Source: CAD feature listing. Evaluate the final solid. Frame: model axes, mm. A direction names the side the tool comes from. Give positions to 0.01 mm unless a question says otherwise; leave off trailing zeros. Order: outer loops, then holes, each group sorted by start corner. A loop starts at its lowest first (then second) coordinate and runs counter-clockwise, first axis right, second up. Notation, with made-up numbers: M 32.5,5 L 74.5,5 A21 ccw 74.5,12 Z; hole C 86,36.5 d7. An arc over 180 degrees is marked long. Answer in a Markdown table with one row per item. Add a question column.
(1) Section query C-C, the plane z = 9. Return loops of the section in (x, y).
(2) Set-up query: faces 1 (the face through (-0.5, 6.5, 4.9)), 2 (the face through (5, 0, 5)). Return all of +Z, -Z, +X, -X, +Y, -Y with unobstructed straight access to the full face (end or side cutting, diameter ignored); none if empty.
(3) Pin query (flat end, axial travel): P1, Ø3, axis at y = 4, z = 4.5, coming from the +X side. Return the tip coordinate at first contact, or that it passes through.
(4) Mould query, pull axis Z, two halves, no side actions, for faces 3 (the face through (-0.507, 3.26, 6.983)), 4 (the face through (-1, 1, 4)). Classes: pulls with the +Z half, pulls with the -Z half, needs draft (parallel to the pull), parting line crosses it, or undercut.
(5) Section query B-B, the plane z = 5. Return loops of the section in (x, y).
(6) Material intervals for line 1 along Z through (x, y) = (-0.7, 3); line 2 along X through (y, z) = (0.25, 2.5), sorted ascending.
(7) Section query A-A, the plane y = 3. Return loops of the section in (x, z).
(8) Section query D-D, the plane y = 4.25. Return loops of the section in (x, z), plus the area to 3 significant figures.
from build123d import *

# Parameters (mm, degrees)
AUFSATZ_LINEAR_AUSTRAGEN1_DEPTH = 10
SKIZZE2_R                       = 2
SCHNITT_LINEAR_AUSTRAGEN1_DEPTH = 16.564382416


with BuildPart() as part:
    # Skizze1 → Aufsatz-Linear austragen1 (new body)
    with BuildSketch(Plane.XY):
        Polygon((0, 0), (0, 6.5), (-1, 6.5), (-1, -1), (9, -1), (9, 0), align=None)
    extrude(amount=AUFSATZ_LINEAR_AUSTRAGEN1_DEPTH)

    # Skizze2 → Schnitt-Linear austragen1 (cut, through all)
    with BuildSketch(Plane.ZY.offset(1)):
        with Locations(Location((5, 3, 0), (0, 0, 270))):
            Circle(SKIZZE2_R)
    extrude(amount=-SCHNITT_LINEAR_AUSTRAGEN1_DEPTH, mode=Mode.SUBTRACT)


solid = part.part
Values follow:
| question | item | result |
|---|---|---|
| 1 | outline | M -1,-1 L 9,-1 L 9,0 L 0,0 L 0,6.5 L -1,6.5 Z |
| 2 | face 1 | +Z, -Z, +X, -X, +Y |
| 2 | face 2 | +Z, -Z, +X, +Y |
| 3 | P1 | stops at x = 0 |
| 4 | face 3 | undercut |
| 4 | face 4 | needs draft |
| 5 | outline | M -1,-1 L 9,-1 L 9,0 L 0,0 L 0,1 L -1,1 Z; M -1,5 L 0,5 L 0,6.5 L -1,6.5 Z |
| 6 | line 1 | z = 0 to 3, 7 to 10 |
| 6 | line 2 | x = -1 to 0 |
| 7 | outline | M -1,0 L 0,0 L 0,3 L -1,3 Z; M -1,7 L 0,7 L 0,10 L -1,10 Z |
| 8 | outline | M -1,0 L 0,0 L 0,3.44 L -1,3.44 Z; M -1,6.56 L 0,6.56 L 0,10 L -1,10 Z |
| 8 | area | 6.88 mm² |
